The model under review builds one solid part; all positions refer to its coordinate system, in mm. Coordinates: 2 decimals unless noted, no trailing zeros. Write each loop counter-clockwise with the first axis right and the second up, starting at its lowest first coordinate (ties: lowest second). Pieces come first, ordered by that corner, then holes.
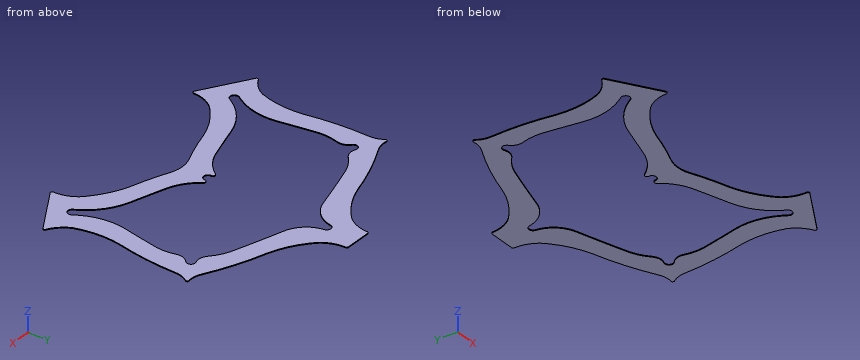
```python
from build123d import *

# Parameters (mm, degrees)
BOSS_EXTRUDE1_DEPTH = 6.35


with BuildPart() as part:
    # Model → Boss-Extrude1 (new body)
    with BuildSketch(Plane.XY):
        with BuildLine():
            Line((-884.322818744, -549.29009194), (-1054.530174704, -445.805078084))
            ThreePointArc((-1054.530174704, -445.805078084), (-1060.015250834, -434.417043276), (-1051.848553213, -424.76932609))
            ThreePointArc((-1051.848553213, -424.76932609), (-985.807567244, -374.734516765), (-939.301155204, -306.163038647))
            ThreePointArc((-939.301155204, -306.163038647), (-905.064557772, -139.536796819), (-912.981608705, 30.386036767))
            ThreePointArc((-912.981608705, 30.386036767), (-947.769666661, 257.241539714), (-958.02502384, 486.519658693))
            ThreePointArc((-958.02502384, 486.519658693), (-965.588685647, 541.638264925), (-990.835960942, 591.214920954))
            ThreePointArc((-990.835960942, 591.214920954), (-991.84055675, 596.69892445), (-990.17277116, 602.018886698))
            ThreePointArc((-990.17277116, 602.018886698), (-986.217231755, 605.947908853), (-980.886171834, 607.57987307))
            ThreePointArc((-980.886171834, 607.57987307), (-925.252472429, 607.981399504), (-872.836959201, 626.633040343))
            ThreePointArc((-872.836959201, 626.633040343), (-664.563021755, 723.046707284), (-447.149449941, 796.565187843))
            ThreePointArc((-447.149449941, 796.565187843), (-319.374365192, 851.948853241), (-205.456380929, 932.05200884))
            ThreePointArc((-205.456380929, 932.05200884), (-182.479274288, 952.925004664), (-160.472351879, 974.818491148))
            ThreePointArc((-160.472351879, 974.818491148), (-120.997454719, 1047.665086581), (-106.969706681, 1129.323621083))
            ThreePointArc((-106.969706681, 1129.323621083), (-104.493884438, 1138.878845883), (-95.559463776, 1143.075051813))
            Line((-95.559463776, 1143.075051813), (0.262323317, 1143.075051813))
            Line((0.262323317, 1143.075051813), (96.08411041, 1143.075051813))
            ThreePointArc((96.08411041, 1143.075051813), (105.018531072, 1138.878845883), (107.494353315, 1129.323621083))
            ThreePointArc((107.494353315, 1129.323621083), (121.522101353, 1047.665086581), (160.996998513, 974.818491148))
            ThreePointArc((160.996998513, 974.818491148), (183.003920922, 952.925004664), (205.981027563, 932.05200884))
            ThreePointArc((205.981027563, 932.05200884), (319.899011826, 851.948853241), (447.674096575, 796.565187843))
            ThreePointArc((447.674096575, 796.565187843), (665.08766839, 723.046707283), (873.361605838, 626.633040341))
            ThreePointArc((873.361605838, 626.633040341), (925.777119065, 607.981399504), (981.410818468, 607.57987307))
            ThreePointArc((981.410818468, 607.57987307), (986.741878389, 605.947908853), (990.697417794, 602.018886698))
            ThreePointArc((990.697417794, 602.018886698), (992.365203384, 596.69892445), (991.360607576, 591.214920954))
            ThreePointArc((991.360607576, 591.214920954), (966.113332281, 541.638264925), (958.549670474, 486.519658693))
            ThreePointArc((958.549670474, 486.519658693), (948.294313295, 257.241539714), (913.506255339, 30.386036768))
            ThreePointArc((913.506255339, 30.386036768), (905.589204406, -139.536796819), (939.825801838, -306.163038647))
            ThreePointArc((939.825801838, -306.163038647), (986.332213878, -374.734516765), (1052.373199847, -424.76932609))
            ThreePointArc((1052.373199847, -424.76932609), (1060.539897468, -434.417043276), (1055.054821338, -445.805078084))
            Line((1055.054821338, -445.805078084), (884.847465378, -549.29009194))
            Line((884.847465378, -549.29009194), (714.640109418, -652.775105795))
            ThreePointArc((714.640109418, -652.775105795), (702.005414591, -652.403779037), (697.19860418, -640.713271323))
            ThreePointArc((697.19860418, -640.713271323), (683.170856142, -559.054736821), (643.695958982, -486.208141388))
            ThreePointArc((643.695958982, -486.208141388), (621.689036573, -464.314654904), (598.711929932, -443.44165908))
            ThreePointArc((598.711929932, -443.44165908), (484.793945672, -363.338503483), (357.018860928, -307.954838085))
            ThreePointArc((357.018860928, -307.954838085), (222.947489099, -265.709568431), (91.944010166, -214.740126023))
            ThreePointArc((91.944010166, -214.740126023), (47.054225612, -200.730515706), (0.262323317, -196.052928909))
            ThreePointArc((0.262323317, -196.052928909), (-46.529578977, -200.730515706), (-91.419363532, -214.740126023))
            ThreePointArc((-91.419363532, -214.740126023), (-222.422842463, -265.70956843), (-356.49421429, -307.954838084))
            ThreePointArc((-356.49421429, -307.954838084), (-484.269299036, -363.338503482), (-598.187283298, -443.44165908))
            ThreePointArc((-598.187283298, -443.44165908), (-621.164389939, -464.314654904), (-643.171312347, -486.208141388))
            ThreePointArc((-643.171312347, -486.208141388), (-682.646209507, -559.054736821), (-696.673957546, -640.713271323))
            ThreePointArc((-696.673957546, -640.713271323), (-701.480767956, -652.403779037), (-714.115462784, -652.775105795))
            Line((-714.115462784, -652.775105795), (-884.322818744, -549.29009194))
        make_face()
        with BuildLine():
            Line((-831.035245163, -400.529794286), (-814.995386538, -374.148178004))
            ThreePointArc((-814.995386538, -374.148178004), (-755.681673534, -217.587288079), (-756.705863237, -50.170503258))
            ThreePointArc((-756.705863237, -50.170503258), (-782.502405832, 88.627483964), (-806.4955468, 227.748553731))
            ThreePointArc((-806.4955468, 227.748553731), (-807.727163724, 299.824157666), (-794.734772679, 370.729780417))
            ThreePointArc((-794.734772679, 370.729780417), (-795.278719619, 421.74664414), (-823.780399516, 464.062959025))
            ThreePointArc((-823.780399516, 464.062959025), (-830.772921751, 505.10476961), (-791.117705256, 517.785045164))
            ThreePointArc((-791.117705256, 517.785045164), (-740.432028836, 511.955939897), (-694.888676898, 534.952012531))
            ThreePointArc((-694.888676898, 534.952012531), (-637.917685406, 579.118919726), (-573.361803176, 611.196133327))
            ThreePointArc((-573.361803176, 611.196133327), (-384.318244806, 670.678328168), (-194.222460106, 726.706812923))
            ThreePointArc((-194.222460106, 726.706812923), (-85.829836181, 794.87078756), (-31.092943269, 910.625532232))
            ThreePointArc((-31.092943269, 910.625532232), (-20.348344787, 929.785400257), (0.262323317, 937.384564654))
            ThreePointArc((0.262323317, 937.384564654), (20.872991421, 929.785400257), (31.617589903, 910.625532232))
            ThreePointArc((31.617589903, 910.625532232), (86.354482821, 794.870787553), (194.747106759, 726.706812918))
            ThreePointArc((194.747106759, 726.706812918), (384.842891449, 670.678328165), (573.886449811, 611.196133327))
            ThreePointArc((573.886449811, 611.196133327), (638.44233204, 579.118919726), (695.413323532, 534.952012531))
            ThreePointArc((695.413323532, 534.952012531), (740.95667547, 511.955939897), (791.642351891, 517.785045164))
            ThreePointArc((791.642351891, 517.785045164), (831.297568385, 505.10476961), (824.30504615, 464.062959025))
            ThreePointArc((824.30504615, 464.062959025), (795.803366253, 421.74664414), (795.259419313, 370.729780417))
            ThreePointArc((795.259419313, 370.729780417), (808.251810359, 299.824157666), (807.020193434, 227.748553731))
            ThreePointArc((807.020193434, 227.748553731), (783.027052467, 88.627483964), (757.230509871, -50.170503258))
            ThreePointArc((757.230509871, -50.170503258), (756.206320168, -217.587288079), (815.520033172, -374.148178004))
            Line((815.520033172, -374.148178004), (831.559891797, -400.529794286))
            ThreePointArc((831.559891797, -400.529794286), (820.925054123, -444.153471661), (777.301376749, -433.518633987))
            Line((777.301376749, -433.518633987), (761.261518123, -407.137017703))
            ThreePointArc((761.261518123, -407.137017703), (649.563377324, -282.425534082), (500.458599124, -206.28622805))
            ThreePointArc((500.458599124, -206.28622805), (365.360989591, -165.310884678), (230.806507684, -122.585783567))
            ThreePointArc((230.806507684, -122.585783567), (135.195604422, -68.689901345), (59.989781623, 11.249420395))
            ThreePointArc((59.989781623, 11.249420395), (42.5119564, 17.019369979), (32.226042951, 1.756124019))
            ThreePointArc((32.226042951, 1.756124019), (23.509796029, -21.903091273), (0.298037309, -31.7491913))
            ThreePointArc((0.298037309, -31.7491913), (0.280180346, -31.749313732), (0.262323317, -31.749426121))
            ThreePointArc((0.262323317, -31.749426121), (0.244466288, -31.749313732), (0.226609326, -31.7491913))
            ThreePointArc((0.226609326, -31.7491913), (-22.985149395, -21.903091273), (-31.701396317, 1.756124019))
            ThreePointArc((-31.701396317, 1.756124019), (-41.987309766, 17.019369979), (-59.465134989, 11.249420395))
            ThreePointArc((-59.465134989, 11.249420395), (-134.670957788, -68.689901345), (-230.28186105, -122.585783567))
            ThreePointArc((-230.28186105, -122.585783567), (-364.836342957, -165.310884677), (-499.93395249, -206.28622805))
            ThreePointArc((-499.93395249, -206.28622805), (-649.038730689, -282.425534082), (-760.736871489, -407.137017703))
            Line((-760.736871489, -407.137017703), (-776.776730114, -433.518633987))
            ThreePointArc((-776.776730114, -433.518633987), (-820.400407489, -444.153471661), (-831.035245163, -400.529794286))
        make_face(mode=Mode.SUBTRACT)
    extrude(amount=BOSS_EXTRUDE1_DEPTH)


solid = part.part
```
Item 1: Take a section at A-A, the plane y = 118. Write out the cut boundary in (x, z), plus the area to 3 significant figures.
Solved:
outline: (-929.38, 0) - (-787.72, 0) - (-787.72, 6.35) - (-929.38, 6.35) - close; (788.25, 0) - (929.91, 0) - (929.91, 6.35) - (788.25, 6.35) - close
area: 1,800 mm2
Item 2: Take a section at B-B, the plane x = -530. Write out the cut boundary in (y, z).
Solved:
outline: (-391.38, 0) - (-216.34, 0) - (-216.34, 6.35) - (-391.38, 6.35) - close; (625.17, 0) - (771.61, 0) - (771.61, 6.35) - (625.17, 6.35) - close
Item 3: For pin 1 (3 mm diameter, centred on x = -460, z = 0.5, fed in from -Y); pin 2 (3 mm diameter, centred on x = 731.5, z = 1.5, fed in from -Y), all flat-tipped, find the tip position at first contact; note any pin that passes through.
Solved:
pin 1: stops at y = -351.13
pin 2: stops at y = -643.44
Item 4: To check wall thickness, follow line 1 along X through (y, z) = (-437.5, 2); line 2 along X through (y, z) = (8, 5.25); line 3 along Y through (x, z) = (-250.5, 2). State the ranges of each line that lie inside material, in increasing order.
Solved:
line 1: x = -1060 to -828.17, -779.64 to -591.25, 591.77 to 780.17, 828.7 to 1060.52
line 2: x = -909.49 to -767.74, -61.73 to -32.67, 33.19 to 62.26, 768.27 to 910.02
line 3: y = -275.36 to -129.13, 710.51 to 896.17
